Verification items for this drawing (mm, ordinates from the low corner). A direction names the side the tool comes from. Round coordinates to 2 decimals unless told otherwise and drop trailing zeros. Order: outer loops, then holes, each group sorted by start corner. A loop starts at its lowest first (then second) coordinate and runs counter-clockwise, first axis right, second up. Notation, with made-up numbers: (77, 59.5) -> (106, 59.5) arc R35 ccw to (106, 98.5) -> close; hole circle Ø2 at (79.5, -1.5). An arc over 180 degrees is marked (long way). Answer in a Markdown table with one row per item. Add a question column.
1. Access from +Z, -Z, +X, -X, +Y, -Y to the whole of each face (thin tool, end or side, straight path). Record for the marked faces 1 and 2.
2. Sectioned sample at C-C, the plane z = 19.5. Record the boundary of the cut face in (x, y).
3. Material ranges on L1, parallel to X at y = 1.2, z = 12.25; L2, parallel to Z at x = 11.5, y = 0.65, recorded low to high. Write a range as from..to.
4. Sectioned sample at B-B, the plane x = 12.25. Record the boundary of the cut face in (y, z), then the cut area to 4 significant figures.
5. Draft check along Z on the marked faces 3, 4, 5 and 6. Enter one of: +Z half, -Z half, draft (parallel to the pull), parting line (faces both ways), or undercut.
6. Depth check by flat-ended pin: P1, Ø2, axis at y = 4, z = 9.5, coming from the -X side. Enter the tip coordinate at first touch or a pass-through.
7. Sectioned sample at D-D, the plane x = 4. Record the boundary of the cut face in (y, z), then the cut area to 3 significant figures.
8. Sectioned sample at A-A, the plane z = 12.25. Record the boundary of the cut face in (x, y).
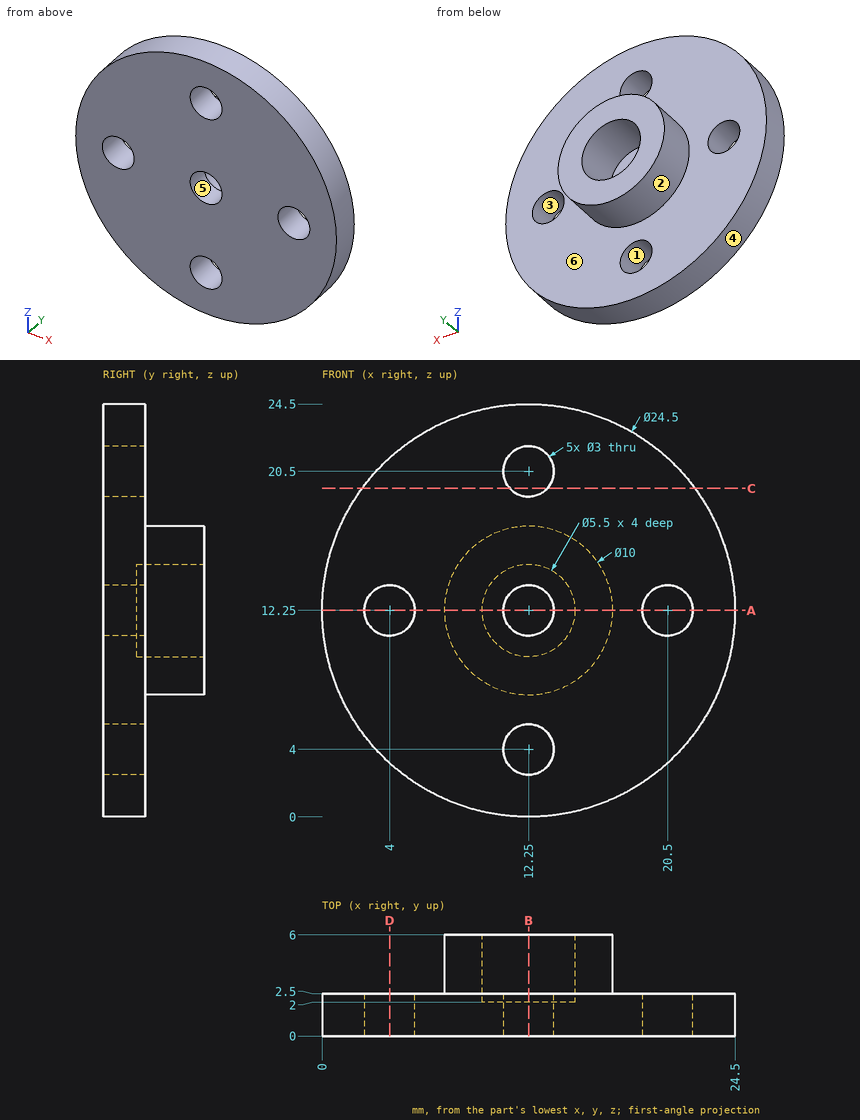
Answer key:
| question | item | result |
|---|---|---|
| 1 | face 1 | +Y, -Y |
| 1 | face 2 | +Y |
| 2 | outline | (2.38, 0) -> (11.13, 0) -> (11.13, 2.5) -> (2.38, 2.5) -> close; (13.37, 0) -> (22.12, 0) -> (22.12, 2.5) -> (13.37, 2.5) -> close |
| 3 | L1 | x = 0..2.5, 5.5..10.75, 13.75..19, 22..24.5 |
| 3 | L2 | z = 0.02..2.7, 5.3..10.95, 13.55..19.2, 21.8..24.48 |
| 4 | outline | (0, 0) -> (2.5, 0) -> (2.5, 2.5) -> (0, 2.5) -> close; (0, 5.5) -> (2.5, 5.5) -> (2.5, 7.25) -> (6, 7.25) -> (6, 9.5) -> (2, 9.5) -> (2, 10.75) -> (0, 10.75) -> close; (0, 13.75) -> (2, 13.75) -> (2, 15) -> (6, 15) -> (6, 17.25) -> (2.5, 17.25) -> (2.5, 19) -> (0, 19) -> close; (0, 22) -> (2.5, 22) -> (2.5, 24.5) -> (0, 24.5) -> close |
| 4 | area | 53.25 mm² |
| 5 | face 3 | undercut |
| 5 | face 4 | parting line |
| 5 | face 5 | undercut |
| 5 | face 6 | draft |
| 6 | P1 | stops at x = 7.57 |
| 7 | outline | (0, 3.19) -> (2.5, 3.19) -> (2.5, 10.75) -> (0, 10.75) -> close; (0, 13.75) -> (2.5, 13.75) -> (2.5, 21.31) -> (0, 21.31) -> close |
| 7 | area | 37.8 mm² |
| 8 | outline | (0, 0) -> (2.5, 0) -> (2.5, 2.5) -> (0, 2.5) -> close; (5.5, 0) -> (10.75, 0) -> (10.75, 2) -> (9.5, 2) -> (9.5, 6) -> (7.25, 6) -> (7.25, 2.5) -> (5.5, 2.5) -> close; (13.75, 0) -> (19, 0) -> (19, 2.5) -> (17.25, 2.5) -> (17.25, 6) -> (15, 6) -> (15, 2) -> (13.75, 2) -> close; (22, 0) -> (24.5, 0) -> (24.5, 2.5) -> (22, 2.5) -> close |
